The model under review builds one solid part; all positions refer to its coordinate system, in mm. Coordinates: 2 decimals unless noted, no trailing zeros. Write each loop counter-clockwise with the first axis right and the second up, starting at its lowest first coordinate (ties: lowest second). Pieces come first, ordered by that corner, then holes.
1) For line 1 (X direction, y = -2.75, z = 1); line 2 (Y direction, x = 23, z = -0.25); line 3 (Z direction, x = 39, y = 0), list the stretches that pass through material, from the lowest coordinate up.
2) Add section C-C, the plane x = 16.5. State the section outline as (y, z) points, then the cut area to 3 significant figures.
3) Mouldability with a two-part tool opening along X and no side actions: class faces 1 (the cylindrical face through (54.845, -1.734, 2.262)), 2 (the cylindrical face through (-12.521, -1.341, 3.233)), 3 (the flat face through (-14, 0, 0)), 4 (the flat face through (-11, 1, 3)) as released by +X, released by -X, zero draft, split by the parting line, or undercut.
4) Add section B-B, the plane y = -2. State the section outline as (x, z) points.
5) For P1, Ø1, axis at x = 19, z = 1, coming from the +Y side; P2, Ø2, axis at x = 40.5, z = -2, coming from the -Y side; P3, Ø1, axis at x = 34.5, z = 2, coming from the +Y side, all flat-tipped, find the tip position at first contact; note any pin that passes through.
6) Add section A-A, the plane z = 0. State the section outline as (x, y) points.
from build123d import *
from build123d.topology import SkipClean

# Parameters (mm, degrees)
SKETCH_2_R          = 3
EXTRUDE_1_DEPTH     = 4
EXTRUDE_2_DEPTH     = 2.5
SKETCH_5_R          = 2.5
EXTRUDE_3_DEPTH     = 9
MIRROR_START        = 15.5
MIRROR_1_DEPTH      = 0.381197772
MIRROR_START_2      = 15.881197772
MIRROR_1_2_DEPTH    = 4.618802228
EXTRUDE_4_DEPTH     = 5
SKETCH_10_R         = 2.5
EXTRUDE_5_DEPTH     = 6
SKETCH_11_R         = 3
EXTRUDE_6_DEPTH     = 5.5
EXTRUDE_START       = 10
SKETCH_12_R         = 3
EXTRUDE_8_DEPTH     = 10
SKETCH_13_R         = 3
EXTRUDE_9_DEPTH     = 10
SKETCH_14_OUTSIDE_W = 32.048
SKETCH_14_OUTSIDE_H = 35.048
SKETCH_14_OUTSIDE_R = 3
CUT_EXTRUDE_2_DEPTH = 59.352377883
SKETCH_15_R         = 3
EXTRUDE_10_DEPTH    = 29.5
EXTRUDE_11_DEPTH    = 26.5
SKETCH_18_R         = 3.5
EXTRUDE_12_DEPTH    = 3
CUT_EXTRUDE_START   = -3
SKETCH_19_R         = 3
SKETCH_19_R_2       = 2.85
CUT_EXTRUDE_3_DEPTH = 0.7


with BuildPart() as part:
    # Sketch 2 → Extrude 1 (new, symmetric)
    with BuildSketch(Plane(origin=(0, 0, 0), x_dir=(0, 0, -1), z_dir=(1, 0, 0))):
        Circle(SKETCH_2_R)
    extrude_1 = extrude(amount=EXTRUDE_1_DEPTH, both=True)

    # Sketch 3 → Extrude 2 (add, symmetric)
    with BuildSketch(Plane(origin=(4, 0, 0), x_dir=(0, 0, -1), z_dir=(1, 0, 0))):
        with BuildLine():
            Line((5, 0), (5, -8))
            ThreePointArc((5, -8), (0, -13), (-5, -8))
            Line((-5, -8), (-5, 0))
            ThreePointArc((-5, 0), (0, 5), (5, 0))
        make_face()
    extrude(amount=EXTRUDE_2_DEPTH, both=True)

    # Cut-Revolve 1: read off the stored shape, not the designer's step
    # Cut-Revolve 1 outline → Cut-Revolve 1 (revolve, cut)
    with BuildSketch(Plane.YX):
        Polygon((13.0002322, 6.118936215), (4.99999958, 1.499999757), (13.0002322, 1.499999757), align=None)
    revolve(axis=Axis((0, 0, 0), (1, 0, 0)), mode=Mode.SUBTRACT)

    # Sketch 5 → Extrude 3 (add)
    with BuildSketch(Plane(origin=(6.5, 0, 0), x_dir=(0, 0, -1), z_dir=(1, 0, 0))):
        with Locations((0, -8)):
            Circle(SKETCH_5_R)
    extrude(amount=EXTRUDE_3_DEPTH)

    # Mirror 1: read off the stored shape, not the designer's step
    # Mirror 1 outline → Mirror 1 (add)
    with BuildSketch(Plane.YZ.offset(MIRROR_START)):
        with BuildLine():
            Line((-8, -5), (0, -5))
            ThreePointArc((0, -5), (5, 0), (0, 5))
            Line((0, 5), (-7.999999997, 5))
            ThreePointArc((-7.999999997, 5), (-13, 2e-09), (-8, -5))
        make_face()
    extrude(amount=MIRROR_1_DEPTH)

    # Mirror 1 2 outline → Mirror 1 2 (add)
    with BuildSketch(Plane.YZ.offset(MIRROR_START_2)):
        with BuildLine():
            Line((-8, -5), (0, -5))
            ThreePointArc((0, -5), (5, 0), (0, 5))
            Line((0, 5), (-7.999999997, 5))
            ThreePointArc((-7.999999997, 5), (-13, 2e-09), (-8, -5))
        make_face()
    extrude(amount=MIRROR_1_2_DEPTH)

    # Mirror 1 3 outline → Mirror 1 3 (revolve, cut)
    with BuildSketch(Plane.YX):
        Polygon((13.0002322, 20.500000243), (4.99999958, 20.500000243), (13.0002322, 15.881063785), align=None)
    revolve(axis=Axis((0, 0, 0), (1, 0, 0)), mode=Mode.SUBTRACT)

    # Mirror 2: Extrude 1 across plane
    add(extrude_1.mirror(Plane(origin=(11, 0, 0), x_dir=(0, 0, 1), z_dir=(1, 0, 0))))

    # Sketch 6 → Extrude 4 (add)
    with BuildSketch(Plane(origin=(26, 0, 0), x_dir=(0, 0, -1), z_dir=(1, 0, 0))):
        with BuildLine():
            Line((0, -5), (-5, -5))
            ThreePointArc((-5, -5), (-10, 0), (-5, 5))
            Line((-5, 5), (0, 5))
            ThreePointArc((0, 5), (5, 0), (0, -5))
        make_face()
    extrude_4 = extrude(amount=EXTRUDE_4_DEPTH)

    # Cut-Revolve 2: read off the stored shape, not the designer's step
    # Cut-Revolve 2 outline → Cut-Revolve 2 (revolve, cut)
    with BuildSketch(Plane.YX):
        Polygon((10.000264544, 30.195720135), (5, 26), (10.000264544, 26), align=None)
    cut_revolve_2 = revolve(axis=Axis((0, 0, 0), (1, 0, 0)), mode=Mode.SUBTRACT)

    # Sketch 10 → Extrude 5 (add)
    with BuildSketch(Plane(origin=(31, 0, 0), x_dir=(0, 0, -1), z_dir=(1, 0, 0))):
        with Locations((-5, 0)):
            Circle(SKETCH_10_R)
    extrude(amount=EXTRUDE_5_DEPTH)

    # Mirror 3: Extrude 4, Cut-Revolve 2 across plane
    add(extrude_4.mirror(Plane(origin=(34, 0, 0), x_dir=(0, 0, 1), z_dir=(1, 0, 0))))
    add(cut_revolve_2.mirror(Plane(origin=(34, 0, 0), x_dir=(0, 0, 1), z_dir=(1, 0, 0))), mode=Mode.SUBTRACT)

    # Sketch 11 → Extrude 6 (add)
    with BuildSketch(Plane(origin=(42, 0, 0), x_dir=(0, 0, -1), z_dir=(1, 0, 0))):
        Circle(SKETCH_11_R)
    extrude(amount=EXTRUDE_6_DEPTH)

    # Sketch 12 → Extrude 8 (add)
    with BuildSketch(Plane.ZY.offset(4).offset(EXTRUDE_START)):
        Circle(SKETCH_12_R)
    extrude(amount=-EXTRUDE_8_DEPTH)

    # Sketch 13 → Extrude 9 (add)
    with BuildSketch(Plane(origin=(47.5, 0, 0), x_dir=(0, 0, -1), z_dir=(1, 0, 0))):
        with Locations(Location((0, 0, 0), (0, 0, 180))):
            Circle(SKETCH_13_R)
    extrude(amount=EXTRUDE_9_DEPTH)

    # Sketch 14 outside → Cut-Extrude 2 (cut, through all)
    with SkipClean():  # the faces are left unmerged after this step: merging them gives an invalid solid
        with BuildSketch(Plane.ZY.offset(-1.5)):
            with Locations((2.5, -4)):
                Rectangle(SKETCH_14_OUTSIDE_W, SKETCH_14_OUTSIDE_H)
            Circle(SKETCH_14_OUTSIDE_R, mode=Mode.SUBTRACT)
        extrude(amount=-CUT_EXTRUDE_2_DEPTH, mode=Mode.SUBTRACT)


with BuildPart() as cut_extrude_2_piece_1:
    # of the separate pieces the step leaves, piece 1, a body of its own (cut_extrude_2_pieces)
    add(part.part.solids().sort_by_distance((37, -1.139901312, 2.775))[0])



with BuildPart() as cut_extrude_2_piece_2:
    # of the separate pieces the step leaves, piece 2, a body of its own (cut_extrude_2_pieces)
    add(part.part.solids().sort_by_distance((6.5, 0, 3))[0])


with BuildPart() as cut_extrude_2_piece_1_1:
    with SkipClean():  # the faces are left unmerged after this step: merging them gives an invalid solid
        add(cut_extrude_2_piece_1.part)

        add(cut_extrude_2_piece_2.part)  # Extrude 10 merges Cut-Extrude 2 piece 2
        # Sketch 15 → Extrude 10 (add)
        with BuildSketch(Plane.ZY.offset(-15.5)):
            Circle(SKETCH_15_R)
        extrude(amount=EXTRUDE_10_DEPTH)

    # Sketch 16 → Extrude 11 (add)
    with BuildSketch(Plane(origin=(31, 0, 0), x_dir=(0, 0, -1), z_dir=(1, 0, 0))):
        with BuildLine():
            ThreePointArc((-2.775, -1.139901312), (-2.5, 0), (-2.775, 1.139901312))
            ThreePointArc((-2.775, 1.139901312), (3, 0), (-2.775, -1.139901312))
        make_face()
    extrude(amount=EXTRUDE_11_DEPTH)

    # Sketch 18 → Extrude 12 (add)
    with BuildSketch(Plane.ZY.offset(14)):
        Circle(SKETCH_18_R)
    extrude(amount=-EXTRUDE_12_DEPTH)

    # Sketch 19 → Cut-Extrude 3 (cut)
    with BuildSketch(Plane(origin=(57.5, 0, 0), x_dir=(0, 0, -1), z_dir=(1, 0, 0)).offset(CUT_EXTRUDE_START)):
        with Locations(Location((0, 0, 0), (0, 0, 180))):
            Circle(SKETCH_19_R)
        Circle(SKETCH_19_R_2, mode=Mode.SUBTRACT)
    extrude(amount=CUT_EXTRUDE_3_DEPTH, mode=Mode.SUBTRACT)


solid = cut_extrude_2_piece_1_1.part
Geometry results:
1. line 1: x = -14 to 54.5, 55.2 to 57.5
1. line 2: y = -2.99 to 2.99
1. line 3: z = -3 to 3
2. outline: circle Ø6 at (0, 0)
2. area: 28.3 mm2
3. face 1: undercut
3. face 2: zero draft
3. face 3: released by -X
3. face 4: released by +X
4. outline: (-14, -2.87) - (-11, -2.87) - (-11, -2.24) - (54.5, -2.24) - (54.5, -2.03) - (55.2, -2.03) - (55.2, -2.24) - (57.5, -2.24) - (57.5, 2.24) - (55.2, 2.24) - (55.2, 2.03) - (54.5, 2.03) - (54.5, 2.24) - (-11, 2.24) - (-11, 2.87) - (-14, 2.87) - close
5. P1: stops at y = 2.96
5. P2: stops at y = -2.83
5. P3: stops at y = 2.6
6. outline: (-14, -3.5) - (-11, -3.5) - (-11, -3) - (54.5, -3) - (54.5, -2.85) - (55.2, -2.85) - (55.2, -3) - (57.5, -3) - (57.5, 3) - (55.2, 3) - (55.2, 2.85) - (54.5, 2.85) - (54.5, 3) - (-11, 3) - (-11, 3.5) - (-14, 3.5) - close
